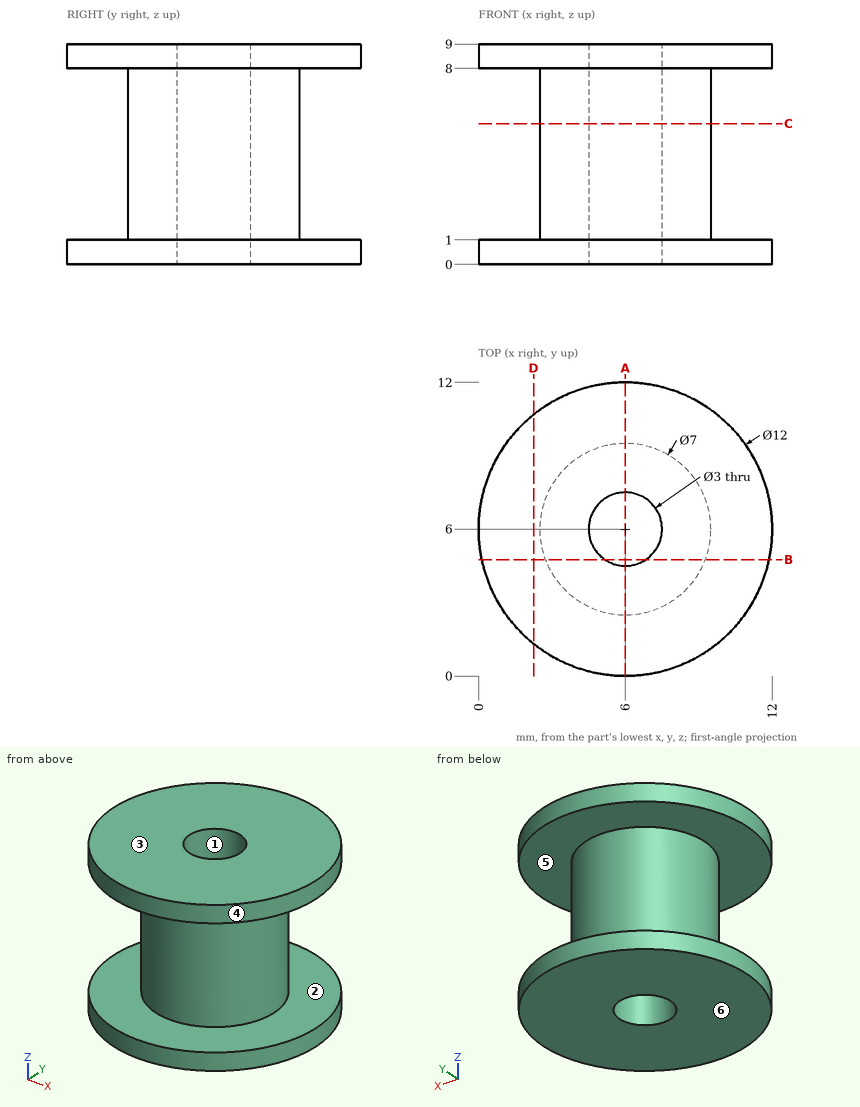
The figure shows three views and two pictorial views of one solid part (mm, origin at its lowest corner). Answer the questions. A direction names the side the tool comes from. Round coordinates to 2 decimals unless told otherwise and drop trailing zeros. Loops run counter-clockwise (first coordinate to the right, second up) from the corner with the lowest first, then second, coordinate; pieces in that order, holes last. Notation, with made-up numbers: (28.5, 39) - (71.5, 39) arc R13 cw to (71.5, 47) - close; hole circle Ø4 at (-12, 38.25). An arc over 180 degrees is marked (long way). One line per question, with ' | ' between items. Start each with the question number.
Q1. Section D-D on x = 2.25 is taken. Give the vertices of the cut face in (y, z).
Q2. Section B-B on y = 4.75 is taken. Give the vertices of the cut face in (x, z).
Q3. Flat-ended cylindrical pins translate along their axes: pin 1 (1 mm diameter, centred on x = 2.5, z = 2, fed in from -Y); pin 2 (6 mm diameter, centred on x = 4.5, y = 6, fed in from -Z); pin 3 (1.5 mm diameter, centred on y = 9.5, z = 3.5, fed in from -X); pin 4 (5 mm diameter, centred on x = 2, z = 8, fed in from -Y). Find the tip coordinate at first contact, or state that the pin passes through.
Q4. For the marked faces 1 and 2, determine the directions among +Z, -Z, +X, -X, +Y, -Y from which every point of the face is accessible in a straight line to the end or side of a thin tool.
Q5. Find the intervals of material crossed by L1, parallel to Y at x = 6, z = 4; L2, parallel to Z at x = 10.75, y = 5.5; L3, parallel to Y at x = 6.5, z = 1.25, in increasing order.
Q6. Section A-A on x = 6 is taken. Give the vertices of the cut face in (y, z).
Q7. For a pull along Z with two mould halves and no side action, classify the marked faces 3, 4, 5 and 6 as +Z half, -Z half, draft (parallel to the pull), parting line (faces both ways), or undercut.
Q8. Section C-C on z = 5.75 is taken. Give the vertices of the cut face in (x, y).
Established:
1) outline: (1.32, 0) - (10.68, 0) - (10.68, 1) - (1.32, 1) - close; (1.32, 8) - (10.68, 8) - (10.68, 9) - (1.32, 9) - close
2) outline: (0.13, 0) - (5.17, 0) - (5.17, 9) - (0.13, 9) - (0.13, 8) - (2.73, 8) - (2.73, 1) - (0.13, 1) - close; (6.83, 0) - (11.87, 0) - (11.87, 1) - (9.27, 1) - (9.27, 8) - (11.87, 8) - (11.87, 9) - (6.83, 9) - close
3) pin 1: y = 4.2 | pin 2: z = 0 | pin 3: x = 3.83 | pin 4: y = 0.19
4) face 1: +Z, -Z | face 2: none
5) L1: 2.5 to 4.5, 7.5 to 9.5 | L2: 0 to 1, 8 to 9 | L3: 2.54 to 4.59, 7.41 to 9.46
6) outline: (0, 0) - (4.5, 0) - (4.5, 9) - (0, 9) - (0, 8) - (2.5, 8) - (2.5, 1) - (0, 1) - close; (7.5, 0) - (12, 0) - (12, 1) - (9.5, 1) - (9.5, 8) - (12, 8) - (12, 9) - (7.5, 9) - close
7) face 3: +Z half | face 4: draft | face 5: undercut | face 6: -Z half
8) outline: circle Ø7 at (6, 6); hole circle Ø3 at (6, 6)
